The listing builds one solid part. Answer for the finished solid, in the listing's coordinates (mm). A direction names the side the tool comes from. Give positions to 0.01 mm unless a question says otherwise; leave off trailing zeros. Loops run counter-clockwise (first coordinate to the right, second up) from the corner with the lowest first, then second, coordinate; pieces in that order, holes last. Notation, with made-up numbers: (-24.5, -29) - (14.5, -29) arc R20 ccw to (14.5, 1) - close; hole circle Ø4 at (9.5, 10). An arc over 180 degrees is marked (long way). Write each question's results on one line, items separated by ' | '.
from build123d import *

# Parameters (mm, degrees)
BUITENAFMETING_RECHTHOEK_W  = 50
BUITENAFMETING_RECHTHOEK_H  = 190
PLAAT_DEPTH                 = 4
TAND_HOR_W                  = 10
TAND_HOR_H                  = 4
TAND_BOVEN_DEPTH            = 5
TANDEN_PATROON_BOVEN_COUNT  = 2
TANDEN_PATROON_BOVEN_PITCH  = 20
TAND_VER_W                  = 4
TAND_VER_H                  = 27.142857143
TAND_LINKS_DEPTH            = 5
TANDEN_PATROON_LINKS_COUNT  = 4
TANDEN_PATROON_LINKS_PITCH  = 54.285714286
TAND_O_W                    = 10
TAND_O_H                    = 4
TAND_ONDER_DEPTH            = 5
TANDEN_PATROON_ONDER_COUNT  = 2
TANDEN_PATROON_ONDER_PITCH  = 20
TAND_R_W                    = 4
TAND_R_H                    = 27.142857143
TAND_RECHTS_DEPTH           = 5
TANDEN_PATROON_RECHTS_COUNT = 4
TANDEN_PATROON_RECHTS_PITCH = 54.285714286


with BuildPart() as part:
    # Buitenafmeting Rechthoek → Plaat (new body)
    with BuildSketch(Plane.XY):
        with Locations((25, 95)):
            Rectangle(BUITENAFMETING_RECHTHOEK_W, BUITENAFMETING_RECHTHOEK_H)
    extrude(amount=-PLAAT_DEPTH)

    # Tand Hor → Tand Boven (cut, through all)
    with BuildSketch(Plane.XY):
        with Locations((15, 188)):
            Rectangle(TAND_HOR_W, TAND_HOR_H)
    tand_boven = extrude(amount=-TAND_BOVEN_DEPTH, mode=Mode.SUBTRACT)

    # Tanden Patroon Boven: Tand Boven ×2
    with Locations(*[(i * TANDEN_PATROON_BOVEN_PITCH, 0, 0) for i in range(1, TANDEN_PATROON_BOVEN_COUNT)]):
        add(tand_boven, mode=Mode.SUBTRACT)

    # Tand Ver → Tand Links (cut, through all)
    with BuildSketch(Plane.XY):
        with Locations((2, 176.428571428)):
            Rectangle(TAND_VER_W, TAND_VER_H)
    tand_links = extrude(amount=-TAND_LINKS_DEPTH, mode=Mode.SUBTRACT)

    # Tanden Patroon Links: Tand Links ×4
    with Locations(*[(0, -i * TANDEN_PATROON_LINKS_PITCH, 0) for i in range(1, TANDEN_PATROON_LINKS_COUNT)]):
        add(tand_links, mode=Mode.SUBTRACT)

    # Tand O → Tand Onder (cut, through all)
    with BuildSketch(Plane.XY):
        with Locations((15, 2)):
            Rectangle(TAND_O_W, TAND_O_H)
    tand_onder = extrude(amount=-TAND_ONDER_DEPTH, mode=Mode.SUBTRACT)

    # Tanden Patroon Onder: Tand Onder ×2
    with Locations(*[(i * TANDEN_PATROON_ONDER_PITCH, 0, 0) for i in range(1, TANDEN_PATROON_ONDER_COUNT)]):
        add(tand_onder, mode=Mode.SUBTRACT)

    # Tand R → Tand Rechts (cut, through all)
    with BuildSketch(Plane.XY):
        with Locations((48, 176.428571428)):
            Rectangle(TAND_R_W, TAND_R_H)
    tand_rechts = extrude(amount=-TAND_RECHTS_DEPTH, mode=Mode.SUBTRACT)

    # Tanden Patroon Rechts: Tand Rechts ×4
    with Locations(*[(0, -i * TANDEN_PATROON_RECHTS_PITCH, 0) for i in range(1, TANDEN_PATROON_RECHTS_COUNT)]):
        add(tand_rechts, mode=Mode.SUBTRACT)


solid = part.part
Item 1: A cutting plane is placed at B-B, the plane y = 78. Determine the outline of the cut face in (x, z).
Values found:
outline: (4, -4) - (46, -4) - (46, 0) - (4, 0) - close
Item 2: Flat-ended cylindrical pins translate along their axes: P1, Ø2, axis at y = 187, z = -2.5, coming from the +X side; P2, Ø2, axis at x = 36.5, z = -1, coming from the -Y side; P3, Ø2, axis at x = 2, z = -1.5, coming from the -Y side. Find the tip coordinate at first contact, or state that the pin passes through.
Values found:
P1: stops at x = 46 | P2: stops at y = 4 | P3: stops at y = 27.14
Item 3: For faces 1 (the face through (15, 186, -2)), 2 (the face through (48, 27.143, -2)), 3 (the face through (10, 2, -2)), 4 (the face through (2, 54.286, -2)), determine the directions among +Z, -Z, +X, -X, +Y, -Y from which every point of the face is accessible in a straight line to the end or side of a thin tool.
Values found:
face 1: +Z, -Z, +Y | face 2: +Z, -Z, +X, -Y | face 3: +Z, -Z, -Y | face 4: +Z, -Z, -X
Item 4: Find the intervals of material crossed by line 1 along Y through (x, z) = (47.5, -0.25); line 2 along Y through (x, z) = (14, -1.65); line 3 along X through (y, z) = (122, -1.9), in increasing order. Write a range as [from, to].
Values found:
line 1: y = [27.14, 54.29], [81.43, 108.57], [135.71, 162.86] | line 2: y = [4, 186] | line 3: x = [4, 46]
Item 5: For a pull along Y with two mould halves and no side action, classify faces 5 (the face through (2, 108.571, -2)), 6 (the face through (7, 0, -2)), 7 (the face through (50, 95, -2)), 8 (the face through (4, 68, -2)) as released by +Y, released by -Y, zero draft, split by the parting line, or undercut.
Values found:
face 5: undercut | face 6: released by -Y | face 7: zero draft | face 8: undercut
Item 6: A cutting plane is placed at A-A, the plane x = 34. Determine the outline of the cut face in (y, z).
Values found:
outline: (4, -4) - (186, -4) - (186, 0) - (4, 0) - close
